from build123d import *

# Parameters (mm, degrees)
SKETCH1_R           = 2.286
SKETCH1_R_2         = 2.032
BOSS_EXTRUDE1_DEPTH = 3.175
CUT_EXTRUDE2_DEPTH  = 112.968585757
FILLET2_R           = 2.54


with BuildPart() as part:
    # Sketch1 → Boss-Extrude1 (new body)
    with BuildSketch(Plane(origin=(0, 0, 0), x_dir=(1, 0, 0), z_dir=(0, 1, 0))):
        with BuildLine():
            Line((-10.998522628, 23.8125), (-14.664696837, 17.4625))
            ThreePointArc((-14.664696837, 17.4625), (-18.565068266, 16.090875015), (-20.514067317, 19.737195774))
            ThreePointArc((-20.514067317, 19.737195774), (-1.724819928, 56.016331719), (32.594151192, 78.184320885))
            ThreePointArc((32.594151192, 78.184320885), (37.76306443, 78.160416217), (41.904450725, 75.06733441))
            Line((41.904450725, 75.06733441), (43.72555591, 72.466526669))
            ThreePointArc((43.72555591, 72.466526669), (44.299748169, 70.645421484), (43.72555591, 68.824316299))
            Line((43.72555591, 68.824316299), (32.798924798, 53.219469855))
            ThreePointArc((32.798924798, 53.219469855), (32.227754435, 51.536856224), (32.650101881, 49.81086467))
            Line((32.650101881, 49.81086467), (53.922601881, 12.965813866))
            Line((53.922601881, 12.965813866), (74.99824615, 3.5308098))
            ThreePointArc((74.99824615, 3.5308098), (79.244408325, -1.084665848), (78.815031546, -7.341513637))
            Line((78.815031546, -7.341513637), (71.755, -21.081542183))
            Line((71.755, -21.081542183), (71.755, -66.675))
            ThreePointArc((71.755, -66.675), (65.736035896, -74.621393426), (56.456352278, -70.979886963))
            Line((56.456352278, -70.979886963), (27.822968614, -24.13))
            Line((27.822968614, -24.13), (27.822968614, -8.73125))
            ThreePointArc((27.822968614, -8.73125), (27.390226607, -5.444248127), (26.121491242, -2.38125))
            Line((26.121491242, -2.38125), (10.998522628, 23.8125))
            ThreePointArc((10.998522628, 23.8125), (0, 30.1625), (-10.998522628, 23.8125))
        make_face()
        with Locations(Location((63.5, -66.675, 0), (0, 0, 270))):
            Circle(SKETCH1_R, mode=Mode.SUBTRACT)
        with Locations(Location((71.755, -3.713861391, 0), (0, 0, 270))):
            Circle(SKETCH1_R_2, mode=Mode.SUBTRACT)
    extrude(amount=BOSS_EXTRUDE1_DEPTH)

    # Sketch4 → Cut-Extrude2 (cut, through all)
    with BuildSketch(Plane(origin=(0, 3.175, 0), x_dir=(1, 0, 0), z_dir=(0, 1, 0))):
        Polygon((38.986058834, -24.13), (62.23, -21.081542183), (62.23, -62.161691573), align=None)
    extrude(amount=-CUT_EXTRUDE2_DEPTH, mode=Mode.SUBTRACT)

    # Fillet2
    fillet2_edges = [part.edges().sort_by_distance(p)[0] for p in [
        (62.23, 1.5875, 62.161691573),
        (38.986058834, 1.5875, 24.13),
        (62.23, 1.5875, 21.081542183),
    ]]
    fillet(fillet2_edges, radius=FILLET2_R)


solid = part.part
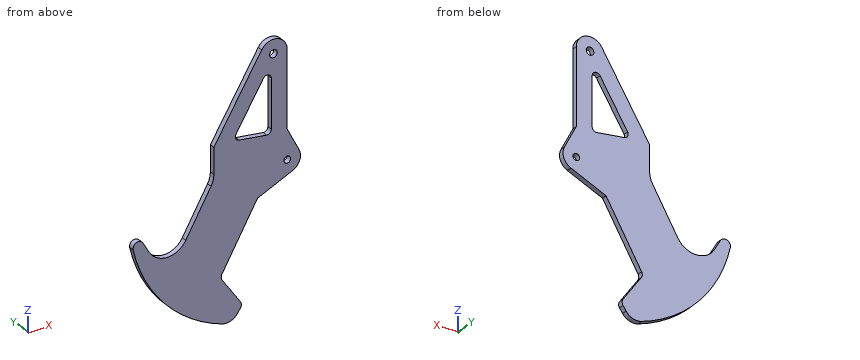
Can you work these out from the model? Positions are in its coordinate system, mm. Give positions to 0.01 mm unless a question says otherwise; leave off trailing zeros. Loops run counter-clockwise (first coordinate to the right, second up) from the corner with the lowest first, then second, coordinate; pieces in that order, holes last. Notation, with made-up numbers: M -36,42 L 5,42 A20 cw 5,54 Z; hole C -21,79.25 d5. An arc over 180 degrees is marked long. One line per item, written item: value.
1) Imagine slicing it at D-D on z = -61. Write out the boundary of the cut face in (x, y) (3 decimals).
Geometry check:
outline: M 3.222,0 L 38.247,0 L 38.247,3.175 L 3.222,3.175 Z
2) I'm going to push flat-ended pins straight in: pin 1 (1.5 mm diameter, centred on x = 60, y = 1.5, fed in from +Z); pin 2 (1.5 mm diameter, centred on y = 0.5, z = -30, fed in from -X); pin 3 (3.5 mm diameter, centred on x = 71.76, z = 3.71, fed in from +Y). Where does each tip first touch, or does it pass through?
Geometry check:
pin 1: stops at z = 74.46
pin 2: stops at x = -17.77
pin 3: passes through
3) Imagine slicing it at C-C on x = 48.5. Write out the boundary of the cut face in (y, z) (3 decimals).
Geometry check:
outline: M 0,-22.358 L 3.175,-22.358 L 3.175,22.882 L 0,22.882 Z; M 0,39.697 L 3.175,39.697 L 3.175,57.962 L 0,57.962 Z
4) Please list where these lines run through material, in increasing order: line 1 (X direction, y = 1.15, z = 65) (3 decimals); line 2 (X direction, y = 2.9, z = 37.5) (3 decimals); line 3 (Z direction, x = -5, y = 0.6).
Geometry check:
line 1: x = 52.802 to 61.944, 65.056 to 71.755
line 2: x = 35.994 to 47.157, 62.23 to 71.755
line 3: z = -52.17 to -29.14
5) Imagine slicing it at B-B on z = 30.5. Write out the boundary of the cut face in (x, y) (3 decimals), and give its area (3 significant figures).
Geometry check:
outline: M 31.716,0 L 42.879,0 L 42.879,3.175 L 31.716,3.175 Z; M 62.23,0 L 71.755,0 L 71.755,3.175 L 62.23,3.175 Z
area: 65.7 mm²
6) Imagine slicing it at A-A on y = 2.05. Count the separate pieces of the cut face and the enclosed holes in it, and give its area (3 significant figures).
Geometry check:
separate pieces: 1
enclosed holes: 3
area: 5,350 mm²
